Geometry: final body of the model. Coordinates: model frame, mm. Give positions to 0.01 mm unless a question says otherwise; leave off trailing zeros. Order: outer loops, then holes, each group sorted by start corner. A loop starts at its lowest first (then second) coordinate and runs counter-clockwise, first axis right, second up. Notation, with made-up numbers: M -19.5,16 L -14.5,16 A20 ccw -14.5,30 Z; hole C 83.25,-21 d5. An arc over 180 degrees is marked long. One line per item, written item: value. Start each with the question number.
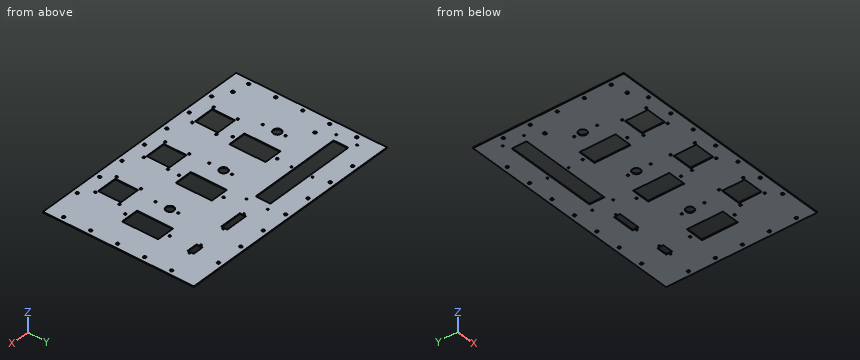
```python
from build123d import *

# Parameters (mm, degrees)
SKETCH_W               = 431.8
SKETCH_H               = 279.4
PAD_DEPTH              = 1.5748
SKETCH002_R            = 1.5875
SKETCH002_W            = 173.95
SKETCH002_H            = 27.45
POCKET_DEPTH           = 1.5758
SKETCH003_R            = 2
SKETCH003_W            = 38.354
SKETCH003_H            = 42.4
POCKET001_DEPTH        = 1.5758
SKETCH004_R            = 2
SKETCH004_R_2          = 7.495
SKETCH004_R_3          = 1.85293
SKETCH004_W            = 33.66
SKETCH004_H            = 67
POCKET002_DEPTH        = 1.5758
SKETCH005_R            = 1.555
SKETCH005_W            = 41.75
SKETCH005_H            = 11.4
POCKET003_DEPTH        = 1.5758
SKETCH006_R            = 1.555
SKETCH006_W            = 20.05
SKETCH006_H            = 11.4
POCKET004_DEPTH        = 1.5758
SKETCH007_R            = 2.61
POCKET005_DEPTH        = 5
LINEARPATTERN_COUNT    = 4
LINEARPATTERN_PITCH    = 50
LINEARPATTERN001_COUNT = 4
LINEARPATTERN001_PITCH = 50
SKETCH008_R            = 2.61
POCKET006_DEPTH        = 1.5758
LINEARPATTERN002_COUNT = 3
LINEARPATTERN002_PITCH = 50
LINEARPATTERN003_COUNT = 3
LINEARPATTERN003_PITCH = 50
SKETCH009_R            = 2.61
POCKET007_DEPTH        = 1.5758
LINEARPATTERN004_COUNT = 4
LINEARPATTERN004_PITCH = 50
LINEARPATTERN005_COUNT = 4
LINEARPATTERN005_PITCH = 50
SKETCH010_R            = 2.61
POCKET008_DEPTH        = 1.5758
LINEARPATTERN006_COUNT = 3
LINEARPATTERN006_PITCH = 50
LINEARPATTERN007_COUNT = 3
LINEARPATTERN007_PITCH = 50
SKETCH011_R            = 2.95
POCKET009_DEPTH        = 1.5758


with BuildPart() as part:
    # Sketch → Pad (new body)
    with BuildSketch(Plane.XY):
        with Locations((0, 139.7)):
            Rectangle(SKETCH_W, SKETCH_H)
    extrude(amount=PAD_DEPTH)

    # Sketch002 → Pocket (cut, through all)
    with BuildSketch(Plane.XY):
        with Locations((-193.025, 243.225)):
            Circle(SKETCH002_R)
        with Locations((6.975, 243.225)):
            Circle(SKETCH002_R)
        with Locations((-193.025, 204.225)):
            Circle(SKETCH002_R)
        with Locations((6.975, 204.225)):
            Circle(SKETCH002_R)
        with Locations((-93.025, 243.225)):
            Circle(SKETCH002_R)
        with Locations((-93.025, 204.225)):
            Circle(SKETCH002_R)
        with Locations((-93.025, 223.725)):
            Rectangle(SKETCH002_W, SKETCH002_H)
    extrude(amount=POCKET_DEPTH, mode=Mode.SUBTRACT)

    # Sketch003 → Pocket001 (cut, through all)
    with BuildSketch(Plane.XY):
        with Locations((-132.229, 72.375)):
            Circle(SKETCH003_R)
        with Locations((-132.229, 27.625)):
            Circle(SKETCH003_R)
        with Locations((-84.479, 27.625)):
            Circle(SKETCH003_R)
        with Locations((-84.479, 72.375)):
            Circle(SKETCH003_R)
        with Locations((-23.875, 72.375)):
            Circle(SKETCH003_R)
        with Locations((23.875, 72.375)):
            Circle(SKETCH003_R)
        with Locations((23.875, 27.625)):
            Circle(SKETCH003_R)
        with Locations((-23.875, 27.625)):
            Circle(SKETCH003_R)
        with Locations((84.479, 72.375)):
            Circle(SKETCH003_R)
        with Locations((132.229, 72.375)):
            Circle(SKETCH003_R)
        with Locations((132.229, 27.625)):
            Circle(SKETCH003_R)
        with Locations((84.479, 27.625)):
            Circle(SKETCH003_R)
        with Locations((-108.354, 50)):
            Rectangle(SKETCH003_W, SKETCH003_H)
        with Locations((0, 50)):
            Rectangle(SKETCH003_W, SKETCH003_H)
        with Locations((108.354, 50)):
            Rectangle(SKETCH003_W, SKETCH003_H)
    extrude(amount=POCKET001_DEPTH, mode=Mode.SUBTRACT)

    # Sketch004 → Pocket002 (cut, through all)
    with BuildSketch(Plane.XY):
        with Locations((-95, 93.75)):
            Circle(SKETCH004_R)
        with Locations((-95, 176.25)):
            Circle(SKETCH004_R)
        with Locations((25, 176.25)):
            Circle(SKETCH004_R)
        with Locations((25, 93.75)):
            Circle(SKETCH004_R)
        with Locations((145, 176.25)):
            Circle(SKETCH004_R)
        with Locations((145, 93.75)):
            Circle(SKETCH004_R)
        with Locations((-145, 135)):
            Circle(SKETCH004_R_2)
        with Locations((-145, 150.48)):
            Circle(SKETCH004_R_3)
        with Locations((-145, 108.32)):
            Circle(SKETCH004_R_3)
        with Locations((-25, 150.48)):
            Circle(SKETCH004_R_3)
        with Locations((-25, 135)):
            Circle(SKETCH004_R_2)
        with Locations((-25, 108.32)):
            Circle(SKETCH004_R_3)
        with Locations((95, 150.48)):
            Circle(SKETCH004_R_3)
        with Locations((95, 135)):
            Circle(SKETCH004_R_2)
        with Locations((95, 108.32)):
            Circle(SKETCH004_R_3)
        with Locations((-95, 135)):
            Rectangle(SKETCH004_W, SKETCH004_H)
        with Locations((25, 135)):
            Rectangle(SKETCH004_W, SKETCH004_H)
        with Locations((145, 135)):
            Rectangle(SKETCH004_W, SKETCH004_H)
    extrude(amount=POCKET002_DEPTH, mode=Mode.SUBTRACT)

    # Sketch005 → Pocket003 (cut, through all)
    with BuildSketch(Plane.XY):
        with Locations((36.55, 224)):
            Circle(SKETCH005_R)
        with Locations((83.45, 224)):
            Circle(SKETCH005_R)
        with Locations((60, 224)):
            Rectangle(SKETCH005_W, SKETCH005_H)
    extrude(amount=POCKET003_DEPTH, mode=Mode.SUBTRACT)

    # Sketch006 → Pocket004 (cut, through all)
    with BuildSketch(Plane.XY):
        with Locations((133.46, 224)):
            Circle(SKETCH006_R)
        with Locations((158.54, 224)):
            Circle(SKETCH006_R)
        with Locations((146, 224)):
            Rectangle(SKETCH006_W, SKETCH006_H)
    extrude(amount=POCKET004_DEPTH, mode=Mode.SUBTRACT)

    # Sketch007 → Pocket005 (cut)
    with BuildSketch(Plane.XY):
        with Locations((0, 9)):
            Circle(SKETCH007_R)
    pocket005 = extrude(amount=POCKET005_DEPTH, mode=Mode.SUBTRACT)

    # LinearPattern: Pocket005 ×4
    with Locations(*[(i * LINEARPATTERN_PITCH, 0, 0) for i in range(1, LINEARPATTERN_COUNT)]):
        add(pocket005, mode=Mode.SUBTRACT)

    # LinearPattern001: Pocket005 ×4
    with Locations(*[(-i * LINEARPATTERN001_PITCH, 0, 0) for i in range(1, LINEARPATTERN001_COUNT)]):
        add(pocket005, mode=Mode.SUBTRACT)

    # Sketch008 → Pocket006 (cut, through all)
    with BuildSketch(Plane.XY):
        with Locations((-206.9, 130.7)):
            Circle(SKETCH008_R)
    pocket006 = extrude(amount=POCKET006_DEPTH, mode=Mode.SUBTRACT)

    # LinearPattern002: Pocket006 ×3
    with Locations(*[(0, -i * LINEARPATTERN002_PITCH, 0) for i in range(1, LINEARPATTERN002_COUNT)]):
        add(pocket006, mode=Mode.SUBTRACT)

    # LinearPattern003: Pocket006 ×3
    with Locations(*[(0, i * LINEARPATTERN003_PITCH, 0) for i in range(1, LINEARPATTERN003_COUNT)]):
        add(pocket006, mode=Mode.SUBTRACT)

    # Sketch009 → Pocket007 (cut, through all)
    with BuildSketch(Plane.XY):
        with Locations((0, 270.4)):
            Circle(SKETCH009_R)
    pocket007 = extrude(amount=POCKET007_DEPTH, mode=Mode.SUBTRACT)

    # LinearPattern004: Pocket007 ×4
    with Locations(*[(i * LINEARPATTERN004_PITCH, 0, 0) for i in range(1, LINEARPATTERN004_COUNT)]):
        add(pocket007, mode=Mode.SUBTRACT)

    # LinearPattern005: Pocket007 ×4
    with Locations(*[(-i * LINEARPATTERN005_PITCH, 0, 0) for i in range(1, LINEARPATTERN005_COUNT)]):
        add(pocket007, mode=Mode.SUBTRACT)

    # Sketch010 → Pocket008 (cut, through all)
    with BuildSketch(Plane.XY):
        with Locations((206.9, 130.7)):
            Circle(SKETCH010_R)
    pocket008 = extrude(amount=POCKET008_DEPTH, mode=Mode.SUBTRACT)

    # LinearPattern006: Pocket008 ×3
    with Locations(*[(0, i * LINEARPATTERN006_PITCH, 0) for i in range(1, LINEARPATTERN006_COUNT)]):
        add(pocket008, mode=Mode.SUBTRACT)

    # LinearPattern007: Pocket008 ×3
    with Locations(*[(0, -i * LINEARPATTERN007_PITCH, 0) for i in range(1, LINEARPATTERN007_COUNT)]):
        add(pocket008, mode=Mode.SUBTRACT)

    # Sketch011 → Pocket009 (cut, through all)
    with BuildSketch(Plane.XY):
        with Locations((-177.8, 177.8)):
            Circle(SKETCH011_R)
        with Locations((-177.8, 25.4)):
            Circle(SKETCH011_R)
    extrude(amount=POCKET009_DEPTH, mode=Mode.SUBTRACT)


with BuildPart() as part_1:
    # Body placement: moved
    add(part.part.moved(Location((-80, -87, -100))))


solid = part_1.part
```
Q1. Section query A-A on y = -26.5. Return loops of the section in (x, z).
Q2. Section query B-B on x = 36. Return loops of the section in (y, z), and give its area (3 significant figures).
Q3. Section query C-C on z = -99.3. Give the number of separate pieces and of enclosed holes in the cut face, and give its area (3 significant figures).
Q4. Ray query, line 1 along Y through (x, z) = (74, -99.05); line 2 along Y through (x, z) = (-257.8, -98.8); line 3 along X through (y, z) = (-38.5, -98.85). Return the intervals inside material, ascending. Write a range as [from, to].
Results below:
1. outline: M -295.9,-100 L -207.53,-100 L -207.53,-98.43 L -295.9,-98.43 Z; M -169.18,-100 L -99.18,-100 L -99.18,-98.43 L -169.18,-98.43 Z; M -60.82,-100 L 9.18,-100 L 9.18,-98.43 L -60.82,-98.43 Z; M 47.53,-100 L 135.9,-100 L 135.9,-98.43 L 47.53,-98.43 Z
2. outline: M -87,-100 L -58.2,-100 L -58.2,-98.43 L -87,-98.43 Z; M -15.8,-100 L 192.4,-100 L 192.4,-98.43 L -15.8,-98.43 Z
2. area: 373 mm2
3. separate pieces: 1
3. enclosed holes: 72
3. area: 102,000 mm2
4. line 1: [-87, 14.5], [81.5, 131.3], [142.7, 192.4]
4. line 2: [-87, -64.55], [-58.65, 87.85], [93.75, 123], [150.45, 192.4]
4. line 3: [-295.9, -207.53], [-169.18, -99.18], [-60.82, 9.18], [47.53, 135.9]
